CAD build for the part. Positions are in the model's coordinates, mm. A direction names the side the tool comes from. Round coordinates to 2 decimals unless told otherwise and drop trailing zeros. Loops run counter-clockwise (first coordinate to the right, second up) from the corner with the lowest first, then second, coordinate; pieces in that order, holes last.
```python
from build123d import *

# Parameters (mm, degrees)
F1_DEPTH = 30.48
F3_DEPTH = 228.601
F5_DEPTH = 355.601


with BuildPart() as f1:
    # F0 (on Top) → F1 (new body)
    with BuildSketch(Plane.XY):
        Polygon((238.922207, -110.560542), (289.722207, -110.560542), (289.722207, 67.239458), (111.922207, 67.239458), (111.922207, 16.439458), (238.922207, 16.439458), align=None)
        Polygon((289.722207, 67.239458), (289.722207, -110.560542), (340.522207, -110.560542), (340.522207, 16.439458), (467.522207, 16.439458), (467.522207, 67.239458), align=None)
        Polygon((111.922207, 67.239458), (289.722207, 67.239458), (238.922207, 118.039458), (111.922207, 118.039458), align=None)
        Polygon((340.522207, 118.039458), (289.722207, 67.239458), (467.522207, 67.239458), (467.522207, 118.039458), align=None)
    extrude(amount=F1_DEPTH)

    # F2 (on face) → F3 (cut, through all)
    with BuildSketch(Plane.XZ.offset(110.560542)):
        Polygon((302.422207, 30.48), (277.022207, 30.48), (289.722207, 17.78), align=None)
    extrude(amount=-F3_DEPTH, mode=Mode.SUBTRACT)

    # F4 (on face) → F5 (cut, through all)
    with BuildSketch(Plane.YZ.offset(467.522207)):
        Polygon((67.239458, 17.78), (79.939458, 30.48), (54.539458, 30.48), align=None)
    extrude(amount=-F5_DEPTH, mode=Mode.SUBTRACT)


solid = f1.part
```
Item 1: 3-axis set-ups, long thin cutter, end or side, ignore diameter. For faces 4 (the flat face through (175, 16.439, 15)), 5 (the flat face through (283.3, -22.9, 24.2)), 6 (the flat face through (202.07, 60.8, 24.22)), 7 (the flat face through (315.48, 93, 15.03)): which of +Z, -Z, +X, -X, +Y, -Y reach the whole face in a straight line?
Answers follow:
face 4: +Z, -Z, -X, -Y
face 5: +Z, +Y, -Y
face 6: +Z, +X, -X
face 7: +Z, -Z, +Y
Item 2: Cut at C-C, the plane x = 164. Give the cut face in (y, z), plus the area to 3 significant figures.
Answers follow:
outline: (16.44, 0) - (118.04, 0) - (118.04, 30.48) - (79.94, 30.48) - (67.24, 17.78) - (54.54, 30.48) - (16.44, 30.48) - close
area: 2,940 mm2
Item 3: Flat gauge pins, fed straight in: P1, Ø9, axis at y = -65, z = 21, coming from the -X side; P2, Ø5, axis at y = 11.5, z = 10, coming from the +X side; P3, Ø15, axis at x = 401.5, z = 15.5, coming from the -Y side; P4, Ø5, axis at y = 62.5, z = 25, coming from the +X side. Where does each tip first touch, or does it go through?
Answers follow:
P1: stops at x = 238.92
P2: stops at x = 340.52
P3: stops at y = 16.44
P4: stops at x = 467.52
Item 4: Two-plate mould, pull along Y, no slides. Class faces 1 (the flat face through (264.68, 92.28, 15.03)), 2 (the flat face through (379.87, 73.5, 24.04)), 3 (the flat face through (238.922, -46, 15)): released by +Y, released by -Y, zero draft, split by the parting line, or undercut.
Answers follow:
face 1: released by +Y
face 2: undercut
face 3: zero draft
Item 5: Probe line 1 (Y direction, x = 450, z = 5); line 2 (X direction, y = -89.5, z = 18.5); line 3 (X direction, y = 80.5, z = 25.5). List the from-to ranges inside material, lowest first.
Answers follow:
line 1: y = 16.44 to 118.04
line 2: x = 238.92 to 289, 290.44 to 340.52
line 3: x = 111.92 to 276.46, 302.98 to 467.52
Item 6: Cut at B-B, the plane z = 22.5. Give the cut face in (x, y), plus the area to 3 significant figures.
Answers follow:
outline: (111.92, 16.44) - (238.92, 16.44) - (238.92, -110.56) - (285, -110.56) - (285, 62.52) - (111.92, 62.52) - close; (111.92, 71.96) - (285, 71.96) - (238.92, 118.04) - (111.92, 118.04) - close; (294.44, -110.56) - (340.52, -110.56) - (340.52, 16.44) - (467.52, 16.44) - (467.52, 62.52) - (294.44, 62.52) - close; (294.44, 71.96) - (467.52, 71.96) - (467.52, 118.04) - (340.52, 118.04) - close
area: 41,500 mm2
Item 7: Cut at A-A, the plane y = -76. Give the cut face in (x, z).
Answers follow:
outline: (238.92, 0) - (340.52, 0) - (340.52, 30.48) - (302.42, 30.48) - (289.72, 17.78) - (277.02, 30.48) - (238.92, 30.48) - close
